Read the model definition and answer for the solid it produces. Units are mm, in the model's axes. Round coordinates to 2 decimals unless told otherwise and drop trailing zeros. Write each loop counter-clockwise with the first axis right and the second up, starting at its lowest first coordinate (ties: lowest second). Pieces come first, ordered by that corner, then holes. Notation, with made-up numbers: (-29.75, 68) - (-11.75, 68) arc R13 cw to (-11.75, 78) - close; hole circle Ø11 at (-21.5, 63). An arc over 180 degrees is marked (long way). Use one line per item in the form item = value. Start each with the question number.
1) The part is cut by section A-A, the plane z = 1. Count the separate pieces of the cut face and the enclosed holes in it, plus the area to 3 significant figures.
2) Consider line 1 along Z through (x, y) = (-103, -4); line 2 along Z through (x, y) = (213, -2). Determine where each line is inside the solid, lowest interval first. Write a range as from..to.
3) The part is cut by section C-C, the plane y = -9.5. Give the vertices of the cut face in (x, z), plus the area to 4 significant figures.
4) The part is cut by section B-B, the plane x = -163. Give the vertices of the cut face in (y, z).
from build123d import *

# Parameters (mm, degrees)
CROQUIS1_W              = 750
CROQUIS1_H              = 40
SALIENTE_EXTRUIR1_DEPTH = 4
CORTAR_EXTRUIR1_DEPTH   = 751
CROQUIS3_R              = 3.96875
CORTAR_EXTRUIR2_DEPTH   = 10


with BuildPart() as part:
    # Croquis1 → Saliente-Extruir1 (new body)
    with BuildSketch(Plane.XY):
        Rectangle(CROQUIS1_W, CROQUIS1_H)
    extrude(amount=SALIENTE_EXTRUIR1_DEPTH)

    # Croquis2 → Cortar-Extruir1 (cut, through all)
    with BuildSketch(Plane(origin=(375, 0, 0), x_dir=(0, 0, -1), z_dir=(1, 0, 0))):
        Polygon((-4, -20), (0, -20), (-4, 0), align=None)
    extrude(amount=-CORTAR_EXTRUIR1_DEPTH, mode=Mode.SUBTRACT)

    # Croquis3 → Cortar-Extruir2 (cut)
    with BuildSketch(Plane(origin=(0, 0, 0), x_dir=(-1, 0, 0), z_dir=(0, 0, -1))):
        with Locations((-350, 12)):
            Circle(CROQUIS3_R)
        with Locations((-300, 12)):
            Circle(CROQUIS3_R)
        with Locations((-250, 12)):
            Circle(CROQUIS3_R)
        with Locations((-200, 12)):
            Circle(CROQUIS3_R)
        with Locations((-150, 12)):
            Circle(CROQUIS3_R)
        with Locations((-100, 12)):
            Circle(CROQUIS3_R)
        with Locations((-50, 12)):
            Circle(CROQUIS3_R)
        with Locations((0, 12)):
            Circle(CROQUIS3_R)
        with Locations((50, 12)):
            Circle(CROQUIS3_R)
        with Locations((100, 12)):
            Circle(CROQUIS3_R)
        with Locations((150, 12)):
            Circle(CROQUIS3_R)
        with Locations((200, 12)):
            Circle(CROQUIS3_R)
        with Locations((250, 12)):
            Circle(CROQUIS3_R)
        with Locations((300, 12)):
            Circle(CROQUIS3_R)
        with Locations((350, 12)):
            Circle(CROQUIS3_R)
    extrude(amount=-CORTAR_EXTRUIR2_DEPTH, mode=Mode.SUBTRACT)


solid = part.part
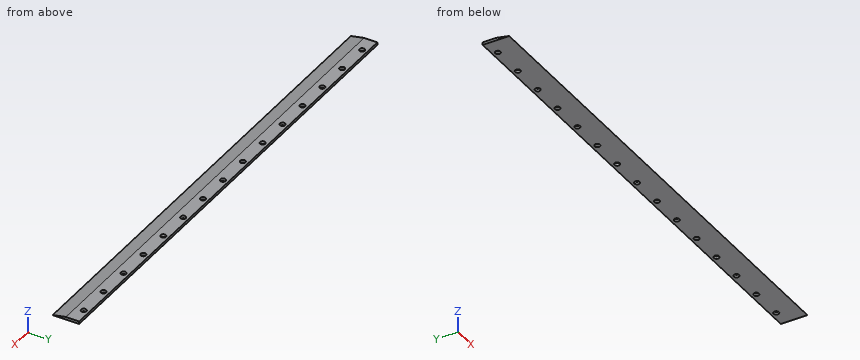
Geometry results:
q1.separate_pieces = 1
q1.enclosed_holes = 15
q1.area = 25,500 mm2
q2.line_1 = 0..3.2
q2.line_2 = 0..3.6
q3.outline = (-375, 0) - (375, 0) - (375, 2.1) - (-375, 2.1) - close
q3.area = 1,575 mm2
q4.outline = (-20, 0) - (20, 0) - (20, 4) - (0, 4) - close
